Geometry: final body of the model. Coordinates: model frame, mm. Face numbers are marked on the shaded views. A direction names the side the tool comes from. Round coordinates to 2 decimals unless told otherwise and drop trailing zeros. Write each loop counter-clockwise with the first axis right and the second up, starting at its lowest first coordinate (ties: lowest second). Pieces come first, ordered by that corner, then holes. Notation, with made-up numbers: M 32,35 L 83,35 A25 cw 83,64 Z; hole C 14.5,-17 d1. An arc over 180 degrees is marked long. Use one line per item in the form item = value. Start each with the question number.
Item 1: Section query B-B (z = -2). Return loops of the section in (x, y), and give its area (3 significant figures).
Item 2: Pin query (flat end, axial travel): pin 1 Ø2 at (x, y) = (7.5, 5) entering from -Z; pin 2 Ø3 at (y, z) = (2, -8) entering from -X; pin 3 Ø20 at (x, z) = (21.28, -8.51) entering from +Y. Return the tip coordinate at first contact, or that it passes through.
Item 3: Reachability of the marked faces 1 and 2 from +Z, -Z, +X, -X, +Y, -Y: full face, straight path, thin tool, end or side. Return the list, or none.
Item 4: Ray query, probe 1 along Z at (x, y) = (15, 3); probe 2 along Z at (x, y) = (18.5, 2.95); probe 3 along Z at (x, y) = (31, 4.55). Return the intervals inside material, ascending.
Item 5: Section query C-C (y = 0.55). Return loops of the section in (x, z).
Item 6: Section query A-A (x = 19). Return loops of the section in (y, z), and give its area (3 significant figures).
Item 7: Pull-direction query (X, two-part tool) for the marked faces 3 and 4; classes: pulls with the +X half, pulls with the -X half, needs draft (parallel to the pull), parting line crosses it, or undercut.
Item 8: Section query D-D (z = -24.5). Return loops of the section in (x, y), and give its area (3 significant figures).
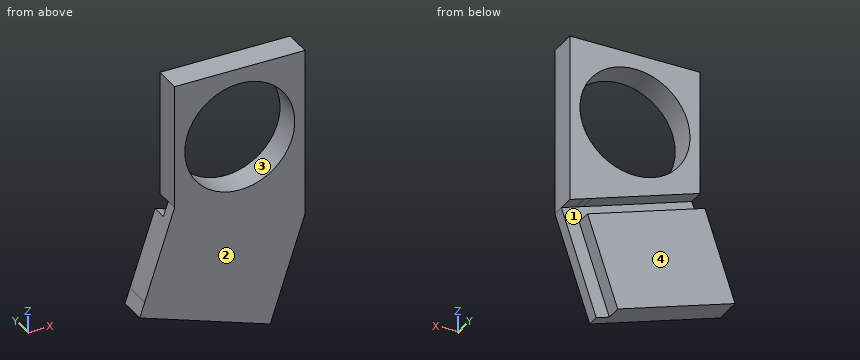
Autodesk Inventor part; units mm, degrees
ref_plane "YZ Plane" through (0, 0, 0) normal (1, 0, 0) x (0, 1, 0)
ref_plane "XZ Plane" through (0, 0, 0) normal (0, 1, 0) x (-1, 0, 0)
ref_plane "XY Plane" through (0, 0, 0) normal (0, 0, 1) x (1, 0, 0)
sketch "Sketch1" plane through (0, 0, 0) normal (0, 1, 0) x (-1, 0, 0)
  line L0 (-8.0312, 5.7806) -> (-34.5277, 5.7806)
  line L1 (-34.5277, 5.7806) -> (-34.5277, -28.5056)
  line L2 (18.6455, 5.0782) -> (18.6456, 5.0782)
  line L3 (-1.974, -37.6808) -> (-8.0312, -19.6194)
  line L4 (-34.5277, -28.5056) -> (-27.4611, -49.5771)
  line L5 (-1.974, -37.6808) -> (-0.9645, -40.691)
  line L6 (-27.4611, -49.5771) -> (-0.9645, -40.691)
  circle A0 centre (-21.2795, -8.5069) radius 11.176
  line L7 (-8.0312, 5.7806) -> (-8.0312, -19.6194)
  line L8 (-8.0312, -19.6194) -> (-0.9645, -40.691)
  line L9 (-0.9645, -40.691) -> (-27.4611, -49.5771)
  line L10 (-27.4611, -49.5771) -> (-34.5277, -28.5056)
  line L11 (-34.5277, -28.5056) -> (-34.5277, 5.7806)
  line L12 (-34.5277, 5.7806) -> (-8.0312, 5.7806)
  point P0 (0, 0)
  dimension "d1" = 22.225
  dimension "d2" = 27.9469
  dimension "d3" = 26.4965
  dimension "d4" = 22.352
  dimension "d20" = 14.2875
  dimension "d23" = 25.4
extrude "Extrusion1" add sketch "Sketch1" along normal blind 5.6134
sketch "Sketch2" plane through (0, 5.6134, 0) normal (0, 1, 0) x (1, 0, 0)
  line L0 (34.5277, 28.5056) -> (8.0312, 19.6194)
  line L1 (8.0312, 19.6194) -> (7.0701, 22.4851)
  line L2 (7.0701, 22.4851) -> (33.5666, 31.3713)
  line L3 (31.5176, 27.4961) -> (29.9884, 26.9832)
  line L4 (34.5277, 28.5056) -> (27.4611, 49.5771)
  point P0 (0, 0)
  point P1 (0, 0)
  dimension "d11" = 3.0226
extrude "Extrusion2" cut sketch "Sketch2" against normal blind 3.175
sketch "Sketch3" plane through (0, 5.6134, 0) normal (0, 1, 0) x (1, 0, 0)
  line L0 (7.0701, 22.4852) -> (33.5666, 31.3713)
  line L1 (33.5666, 31.3713) -> (27.4611, 49.5771)
  line L2 (27.4611, 49.5771) -> (0.9645, 40.691)
  line L3 (24.8, 48.6846) -> (30.9056, 30.4789)
  point P0 (0, 0)
  dimension "d17" = 2.8067
extrude "Extrusion3" cut sketch "Sketch3" against normal blind 3.175
properties part number "Lidar Sensor Case Piece 2"
Working result:
q1.outline = M 8.03,0 L 12.19,0 L 12.19,5.61 L 8.03,5.61 Z; M 30.37,0 L 34.53,0 L 34.53,5.61 L 30.37,5.61 Z
q1.area = 46.7 mm²
q2.pin_1 = -43.22
q2.pin_2 = 8.03
q2.pin_3 = through
q3.face_1 = +Y
q3.face_2 = +Z, -Z, +X, -X, -Y
q4.probe_1 = -45.4 to -25.14, -21.96 to -17.75, 0.74 to 5.78
q4.probe_2 = -46.57 to -26.32, -23.13 to -19.33, 2.32 to 5.78
q4.probe_3 = -27.32 to -14.02, -2.99 to 5.78
q5.outline = M 0.96,-40.69 L 27.46,-49.58 L 34.53,-28.51 L 34.53,5.78 L 8.03,5.78 L 8.03,-19.62 L 1.97,-37.68 Z; hole C 21.28,-8.51 d22.35
q6.outline = M 0,-46.74 L 5.61,-46.74 L 5.61,-26.49 L 2.44,-26.49 L 2.44,-23.3 L 5.61,-23.3 L 5.61,-19.45 L 0,-19.45 Z; M 0,2.43 L 5.61,2.43 L 5.61,5.78 L 0,5.78 Z
q6.area = 162 mm²
q7.face_3 = undercut
q7.face_4 = needs draft
q8.outline = M 6.39,0 L 34.53,0 L 34.53,5.61 L 22.58,5.61 L 22.58,2.44 L 13.08,2.44 L 13.08,5.61 L 6.39,5.61 Z
q8.area = 128 mm²
